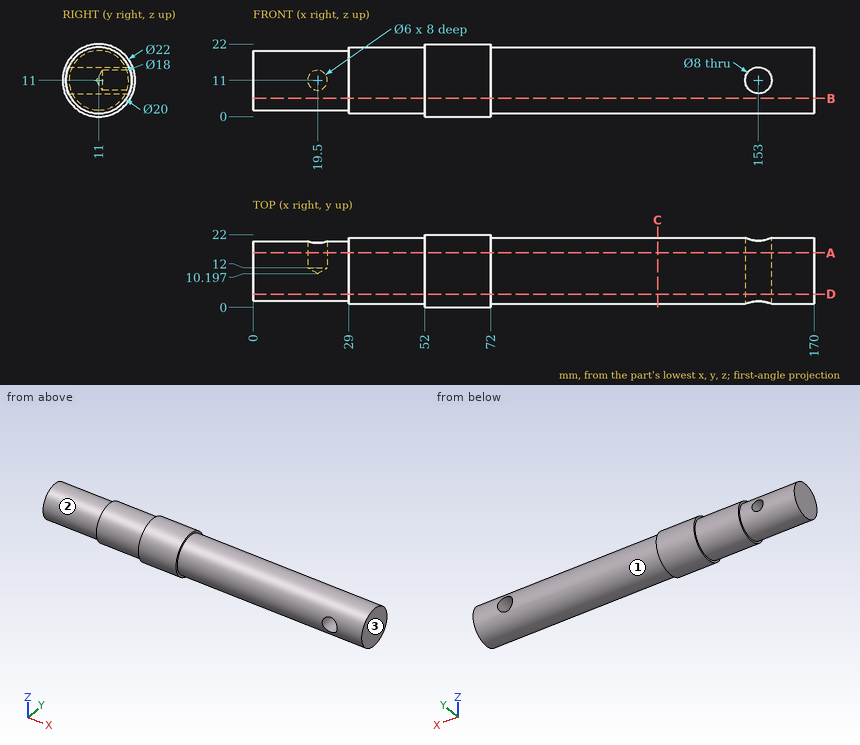
Here's the drawing with two shaded views (mm, measured from the low corner). I have some questions. A direction names the side the tool comes from. Coordinates: 2 decimals unless noted, no trailing zeros. Loops run counter-clockwise (first coordinate to the right, second up) from the corner with the lowest first, then second, coordinate; pieces in that order, holes last. Notation, with made-up numbers: M 59,-37 L 65,-37 A4 ccw 65,-33 Z; hole C 60.25,2 d8. An arc over 180 degrees is marked long. Answer as CSV lines item,"result". Start each with the question number.
1. For pin 1 Ø2 at (x, y) = (119.5, 14.5) entering from -Z; pin 2 Ø5.5 at (x, z) = (19.5, 11) entering from -Y; pin 3 Ø10 at (x, y) = (146, 8) entering from -Z, each with a flat end and sliding along its axis, tell me the tip position at first contact or that it passes through.
2. Suppose I cut it at A-A, the plane y = 16.5. List the corners of the cut face in (x, z) for me.
3. Suppose I cut it at B-B, the plane z = 5.5. List the corners of the cut face in (x, y) for me, plus the area to 3 significant figures.
4. Suppose I cut it at D-D, the plane y = 4. List the corners of the cut face in (x, z) for me (1 decimal), plus the area to 3 significant figures.
5. Suppose I cut it at C-C, the plane x = 122.5. List the corners of the cut face in (y, z) for me.
6. For the marked faces 1, 2 and 3, which set-ups out of +Z, -Z, +X, -X, +Y, -Y let a thin tool reach every point of the face, with its end or its side?
7. If I drill on probe 1 along X at (y, z) = (16.5, 11); probe 2 along Z at (x, y) = (153, 10.5); probe 3 along X at (y, z) = (4.25, 11.25), over which ranges is the centre line in solid material (lowest first)? Write a range as [from, to].
Output:
1,pin 1,"stops at z = 1.32"
1,pin 2,"stops at y = 2"
1,pin 3,"stops at z = 1"
2,outline,"M 0,3.88 L 29,3.88 L 29,2.65 L 52,2.65 L 52,1.47 L 72,1.47 L 72,2.65 L 170,2.65 L 170,19.35 L 72,19.35 L 72,20.53 L 52,20.53 L 52,19.35 L 29,19.35 L 29,18.12 L 0,18.12 Z; hole C 19.5,11 d6; hole C 153,11 d8"
3,outline,"M 0,3.88 L 29,3.88 L 29,2.65 L 52,2.65 L 52,1.47 L 72,1.47 L 72,2.65 L 170,2.65 L 170,19.35 L 72,19.35 L 72,20.53 L 52,20.53 L 52,19.35 L 29,19.35 L 29,18.12 L 0,18.12 Z"
3,area,"2,820 mm^2"
4,outline,"M 0,5.3 L 29,5.3 L 29,3.9 L 52,3.9 L 52,2.5 L 72,2.5 L 72,3.9 L 170,3.9 L 170,18.1 L 72,18.1 L 72,19.5 L 52,19.5 L 52,18.1 L 29,18.1 L 29,16.7 L 0,16.7 Z; hole C 153,11 d8"
4,area,"2,350 mm^2"
5,outline,"C 11,11 d20"
6,face 1,"+X"
6,face 2,"-X"
6,face 3,"+Z, -Z, +X, +Y, -Y"
7,probe 1,"x = [0, 16.5], [22.5, 149], [157, 170]"
7,probe 2,"z = [1.01, 7], [15, 20.99]"
7,probe 3,"x = [0, 149.01], [156.99, 170]"
